Design review of the part built by this model. Coordinates are the model's own, in mm. Face numbers are marked on the shaded views. A direction names the side the tool comes from. Coordinates: 2 decimals unless noted, no trailing zeros. Write each loop counter-clockwise with the first axis right and the second up, starting at its lowest first coordinate (ties: lowest second). Pieces come first, ordered by that corner, then holes.
Q1. Take a section at D-D (x = 10). Give the boundary of the cut face in (y, z), and give its area (3 significant figures).
Q2. Insertion check: pin 1 (5 mm diameter, centred on x = 3.5, y = 26, fed in from +Z); pin 2 (3 mm diameter, centred on x = 6, y = 25.25, fed in from -Z); pin 3 (3 mm diameter, centred on x = 1.5, y = 0, fed in from +Z). Each pin has a flat end and moves straight along its axis. Give the tip position at first contact, or say it passes through.
Q3. Take a section at A-A (y = 11). Give the boundary of the cut face in (x, z).
Q4. For probe 1 along X at (y, z) = (-2.25, 17.1) (3 decimals); probe 2 along Y at (x, z) = (7, 7.25); probe 3 along Z at (x, y) = (8.25, 10), list the stretches that pass through material, from the lowest coordinate up.
Q5. Take a section at B-B (x = 4.5). Give the boundary of the cut face in (y, z), and give its area (3 significant figures).
Q6. Take a section at C-C (z = 27). Give the boundary of the cut face in (x, y) (3 decimals), and give its area (3 significant figures).
Q7. Machinability: for the marked faces 1, 2, 3, 4 and 5, which of the approach directions +Z, -Z, +X, -X, +Y, -Y give a long, thin tool a straight path to every point of the face, cutting with its end or side? Answer none if there is none.
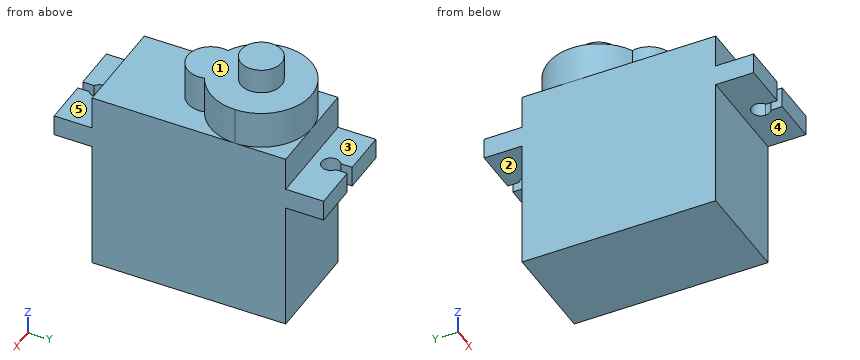
```python
from build123d import *

# Parameters (mm, degrees)
F0_W      = 12
F0_H      = 23
F1_DEPTH  = 22
F3_W      = 12
F3_H      = 4.5
F4_DEPTH  = 2.5
F6_DEPTH  = 18.001
F8_DEPTH  = 4.5
F9_R      = 2.425
F10_DEPTH = 3


with BuildPart() as f1:
    # F0 (on Top) → F1 (new body)
    with BuildSketch(Plane.XY):
        with Locations((6, 11.5)):
            Rectangle(F0_W, F0_H)
    extrude(amount=F1_DEPTH)

    # F3 (on offset) → F4 (join)
    with BuildSketch(Plane.XY.offset(15.5)):
        with Locations((6, 25.25)):
            Rectangle(F3_W, F3_H)
        with Locations((6, -2.25)):
            Rectangle(F3_W, F3_H)
    extrude(amount=F4_DEPTH)

    # F5 (on face) → F6 (cut, through all)
    with BuildSketch(Plane.XY.offset(18)):
        with BuildLine():
            ThreePointArc((5.425, 26.158295), (5.481589, 24.30826), (7.075, 25.25))
            ThreePointArc((7.075, 25.25), (6.94174, 25.768411), (6.575, 26.158295))
            ThreePointArc((6.575, 26.158295), (6, 26.325), (5.425, 26.158295))
        make_face()
        with BuildLine():
            ThreePointArc((5.425, 26.158295), (6, 26.325), (6.575, 26.158295))
            Line((6.575, 26.158295), (6.575, 27.5))
            Line((6.575, 27.5), (5.425, 27.5))
            Line((5.425, 27.5), (5.425, 26.158295))
        make_face()
        with BuildLine():
            Line((5.425, -4.5), (6.575, -4.5))
            Line((6.575, -4.5), (6.575, -3.158295))
            ThreePointArc((6.575, -3.158295), (6, -3.325), (5.425, -3.158295))
            Line((5.425, -3.158295), (5.425, -4.5))
        make_face()
        with BuildLine():
            ThreePointArc((5.425, -3.158295), (6, -3.325), (6.575, -3.158295))
            ThreePointArc((6.575, -3.158295), (6.94174, -2.768411), (7.075, -2.25))
            ThreePointArc((7.075, -2.25), (5.481589, -1.30826), (5.425, -3.158295))
        make_face()
    extrude(amount=-F6_DEPTH, mode=Mode.SUBTRACT)

    # F7 (on face) → F8 (join)
    with BuildSketch(Plane.XY.offset(22)):
        with BuildLine():
            ThreePointArc((8.676815, 11.630208), (11.102004, 13.84254), (12, 17))
            ThreePointArc((12, 17), (2.84254, 22.102004), (3.323185, 11.630208))
            ThreePointArc((3.323185, 11.630208), (6, 11), (8.676815, 11.630208))
        make_face()
        with BuildLine():
            ThreePointArc((8.676815, 11.630208), (6, 11), (3.323185, 11.630208))
            ThreePointArc((3.323185, 11.630208), (6, 8.25), (8.676815, 11.630208))
        make_face()
    extrude(amount=F8_DEPTH)

    # F9 (on face) → F10 (join)
    with BuildSketch(Plane.XY.offset(26.5)):
        with Locations((6, 17)):
            Circle(F9_R)
    extrude(amount=F10_DEPTH)


solid = f1.part
```
Response:
1. outline: (-4.5, 15.5) - (0, 15.5) - (0, 0) - (23, 0) - (23, 15.5) - (27.5, 15.5) - (27.5, 18) - (23, 18) - (23, 22) - (21.47, 22) - (21.47, 26.5) - (12.53, 26.5) - (12.53, 22) - (0, 22) - (0, 18) - (-4.5, 18) - close
1. area: 569 mm2
2. pin 1: stops at z = 18
2. pin 2: stops at z = 15.5
2. pin 3: stops at z = 22
3. outline: (0, 0) - (12, 0) - (12, 22) - (8.75, 22) - (8.75, 26.5) - (3.25, 26.5) - (3.25, 22) - (0, 22) - close
4. probe 1: x = 0 to 4.925, 7.075 to 12
4. probe 2: y = 0 to 23
4. probe 3: z = 0 to 26.5
5. outline: (-4.5, 15.5) - (0, 15.5) - (0, 0) - (23, 0) - (23, 15.5) - (27.5, 15.5) - (27.5, 18) - (23, 18) - (23, 22) - (22.81, 22) - (22.81, 26.5) - (18.91, 26.5) - (18.91, 29.5) - (15.09, 29.5) - (15.09, 26.5) - (8.7, 26.5) - (8.7, 22) - (0, 22) - (0, 18) - (-4.5, 18) - close
5. area: 603 mm2
6. outline: circle Ø4.85 at (6, 17)
6. area: 18.5 mm2
7. face 1: +Z
7. face 2: -Z, +X, -X, +Y
7. face 3: +Z, +X, -X, +Y
7. face 4: -Z, +X, -X, -Y
7. face 5: +Z, +X, -X, -Y
